Input: part model. Units: mm. Frame: model coordinates. A direction names the side the tool comes from. Coordinates: 2 decimals unless noted, no trailing zeros. Loops run counter-clockwise (first coordinate to the right, second up) from the corner with the lowest first, then second, coordinate; pieces in that order, holes last.
(1) Contact query for flat-ended pins moving along their axis: P1, Ø0.9, axis at x = 0, z = 0.5, coming from the -Y side; P2, Ø1.5, axis at y = 8.5, z = -6.5, coming from the -X side; P3, Ø1, axis at x = -1, y = 6.5, coming from the +Z side; P4, Ø5, axis at x = -2, y = 10, coming from the -Z side. Output: stop coordinate, or through.
(2) Line query: L1, parallel to Z at x = 0, y = 2.75; L2, parallel to X at y = 1, z = 4.25; L3, parallel to Z at x = 4, y = 6.25. Output: solid intervals per line, ascending.
(3) Mould query, pull axis X, two halves, no side actions, for faces 3 (the face through (1.172, 4.93, -8.923)), 4 (the face through (-3, 0, -6)), 5 (the face through (5.158, 3.944, 3.955)). Classes: released by +X, released by -X, zero draft, split by the parting line, or undercut.
(4) Section A-A, the plane y = 1.5. Return loops of the section in (x, z), then the cut area to 3 significant figures.
(5) Set-up query: faces 1 (the face through (0, 13, 0)), 2 (the face through (0, 15, 0)). Return all of +Z, -Z, +X, -X, +Y, -Y with unobstructed straight access to the full face (end or side cutting, diameter ignored); none if empty.
Autodesk Inventor part; units mm, degrees
ref_plane "YZ Plane" through (0, 0, 0) normal (1, 0, 0) x (0, 1, 0)
ref_plane "XZ Plane" through (0, 0, 0) normal (0, 1, 0) x (-1, 0, 0)
ref_plane "XY Plane" through (0, 0, 0) normal (0, 0, 1) x (1, 0, 0)
sketch "스케치1" plane through (0, 0, 0) normal (0, 1, 0) x (-1, 0, 0)
  circle A0 centre (0, 0) radius 6.5
  circle A1 centre (0, 0) radius 9
  dimension "d0" = 13
  dimension "d1" = 18
extrude "돌출1" add sketch "스케치1" along normal blind 13
sketch "스케치2" plane through (0, 13, 0) normal (0, 1, 0) x (1, 0, 0)
  circle A0 centre (0, 0) radius 9
  circle A1 centre (0, 0) radius 6.5
extrude "돌출2" add sketch "스케치2" along normal blind 2 contours A0 | A1
fillet "모깎기1" radius 5 2 edges at (6.5, 13, 0) (-9, 15, 0)
thread "스레드1"
properties part number "부품1"
Report:
1. P1: stops at y = 13
1. P2: stops at x = -6.92
1. P3: stops at z = 8.99
1. P4: stops at z = -9
2. L1: z = -9 to -6.5, 6.5 to 9
2. L2: x = -7.93 to -4.92, 4.92 to 7.93
2. L3: z = -8.06 to -5.12, 5.12 to 8.06
3. face 3: split by the parting line
3. face 4: zero draft
3. face 5: undercut
4. outline: circle Ø18 at (0, 0); hole circle Ø13 at (0, 0)
4. area: 122 mm2
5. face 1: -Y
5. face 2: +Z, -Z, +X, -X, +Y
